```python
from build123d import *

# Parameters (mm, degrees)
CHAMFER1_SIZE      = 0.625
CHAMFER2_SIZE      = 0.315
CUT_EXTRUDE3_DEPTH = 2.25


with BuildPart() as part:
    # Sketch1 → Revolve1 (revolve)
    with BuildSketch(Plane(origin=(0, 0, 0), x_dir=(0, 0, -1), z_dir=(1, 0, 0)), mode=Mode.PRIVATE) as revolve1_sk:
        Polygon((0, 5), (4.5, 5), (4.5, 3), (20.5, 3), (20.5, 2.5), (30.5, 2.5), (30.5, 0), (0, 0), align=None)
    revolve(revolve1_sk.sketch.rotate(Axis((0, 0, -30.5), (0, 0, 1)), 90), axis=Axis((0, 0, -30.5), (0, 0, 1)))

    # Sketch5 → Cut-Revolve1 (revolve, cut)
    with BuildSketch(Plane(origin=(0, 0, 0), x_dir=(0, 0, -1), z_dir=(1, 0, 0)), mode=Mode.PRIVATE) as cut_revolve1_sk:
        with BuildLine():
            Line((20.5, 3), (24.250000008, 3))
            Line((24.250000008, 3), (23, 1.749999993))
            Line((23, 1.749999993), (21.250000008, 1.749999993))
            ThreePointArc((21.250000008, 1.749999993), (20.719669916, 1.969669909), (20.5, 2.5))
            Line((20.5, 2.5), (20.5, 3))
        make_face()
    revolve(cut_revolve1_sk.sketch.rotate(Axis((0, 0, -30.5), (0, 0, 1)), 90), axis=Axis((0, 0, -30.5), (0, 0, 1)), mode=Mode.SUBTRACT)

    # Chamfer1
    chamfer1_edges = [part.edges().sort_by_distance(p)[0] for p in [
        (2.5, 0, -30.5),
    ]]
    chamfer(chamfer1_edges, length=CHAMFER1_SIZE)

    # Chamfer2
    chamfer2_edges = [part.edges().sort_by_distance(p)[0] for p in [
        (3, 0, -20.5),
        (5, 0, 0),
    ]]
    chamfer(chamfer2_edges, length=CHAMFER2_SIZE)

    # Sketch8 → Cut-Extrude3 (cut)
    with BuildSketch(Plane.XY):
        Polygon((1.5, 0.866025404), (0, 1.732050808), (-1.5, 0.866025404), (-1.5, -0.866025404), (0, -1.732050808), (1.5, -0.866025404), align=None)
    extrude(amount=-CUT_EXTRUDE3_DEPTH, mode=Mode.SUBTRACT)

    # Cut-Extrude4 cone 1 section (on through the dimple's axis) → Cut-Extrude4 (revolve, cut)
    with BuildSketch(Plane(origin=(0, 0, 0), x_dir=(0, -1, 0), z_dir=(1, 0, 0))):
        Polygon((0, 0), (1.732050808, 0), (0, 1.732050808), align=None)
    revolve(axis=Axis((0, 0, 0), (0, 0, -1)), mode=Mode.SUBTRACT)


solid = part.part
```
Input: part model. Units: mm. Frame: model coordinates. A direction names the side the tool comes from. Give positions to 0.01 mm unless a question says otherwise; leave off trailing zeros. Order: outer loops, then holes, each group sorted by start corner. A loop starts at its lowest first (then second) coordinate and runs counter-clockwise, first axis right, second up. Notation, with made-up numbers: (62.25, 16.5) - (106.25, 16.5) arc R19 ccw to (106.25, 45.5) - close; hole circle Ø4 at (78, 25.25). An arc over 180 degrees is marked (long way). One line per item, written item: value.
1. Line query: probe 1 along Z at (x, y) = (-2.75, -2.75); probe 2 along Z at (x, y) = (1.25, 0); probe 3 along X at (y, z) = (1.5, -21). Output: solid intervals per line, ascending.
Determined:
probe 1: -4.5 to 0
probe 2: -30.5 to -2.25
probe 3: -0.98 to 0.98
2. Draft query along Y for faces 1 (the face through (-2.86, -0.9, -12.45)), 2 (the face through (0.74, -1.305, -1.109)), 3 (the face through (0, 0, -30.5)). Return one class per face: released by +Y, released by -Y, zero draft, split by the parting line, or undercut.
Determined:
face 1: split by the parting line
face 2: undercut
face 3: zero draft
3. Cut plane C-C, the plane z = -9.5. Output: boundary loops of the cut face in (x, y).
Determined:
outline: circle Ø6 at (0, 0)
4. Pin query (flat end, axial travel): pin 1 Ø5 at (y, z) = (-3, -12) entering from +X; pin 2 Ø1.5 at (x, y) = (0, 0.5) entering from +Z; pin 3 Ø1 at (x, z) = (-3, -13) entering from -Y. Return the tip coordinate at first contact, or that it passes through.
Determined:
pin 1: x = 2.96
pin 2: z = -2.25
pin 3: y = -1.66
5. Cut plane B-B, the plane z = -27. Output: boundary loops of the cut face in (x, y), and give its area (3 significant figures).
Determined:
outline: circle Ø5 at (0, 0)
area: 19.6 mm2
6. Reachability of faces 4 (the face through (5, 0, -2)), 5 (the face through (-3.3, -0.1, -4.5)), 6 (the face through (-0.761, -1.293, -1.109)), 7 (the face through (-0.81, 1.55, -22.11)) from +Z, -Z, +X, -X, +Y, -Y: full face, straight path, thin tool, end or side. Return the list, or none.
Determined:
face 4: +Z, -Z
face 5: -Z
face 6: +Z
face 7: none
